Check sheet for the modelled part. Datum: model origin and axes. Units: mm. A direction names the side the tool comes from. Give positions to 0.01 mm unless a question says otherwise; leave off trailing zeros. Order: outer loops, then holes, each group sorted by start corner. A loop starts at its lowest first (then second) coordinate and runs counter-clockwise, first axis right, second up.
from build123d import *

# Parameters (mm, degrees)
SKETCH1_W           = 25
SKETCH1_H           = 25
SKETCH1_W_2         = 20
SKETCH1_H_2         = 20
BOSS_EXTRUDE1_DEPTH = 45
BOSS_EXTRUDE4_DEPTH = 45
FILLET2_R           = 2


with BuildPart() as part:
    # Sketch1 → Boss-Extrude1 (new body)
    with BuildSketch(Plane(origin=(0, 0, 0), x_dir=(1, 0, 0), z_dir=(0, 1, 0))):
        with Locations((12.5, 12.5)):
            Rectangle(SKETCH1_W, SKETCH1_H)
        with Locations((12.5, 12.5)):
            Rectangle(SKETCH1_W_2, SKETCH1_H_2, mode=Mode.SUBTRACT)
    extrude(amount=BOSS_EXTRUDE1_DEPTH)

    # Sketch3 → Boss-Extrude4 (add, through all)
    with BuildSketch(Plane.XZ):
        Polygon((22.5, -2.5), (12.5, -23.5), (2.5, -2.5), (4.404761905, -2.5), (12.5, -19.5), (20.595238095, -2.5), align=None)
    extrude(amount=-BOSS_EXTRUDE4_DEPTH)

    # Fillet2
    fillet2_edges = [part.edges().sort_by_distance(p)[0] for p in [
        (2.5, 22.5, -22.5),
        (22.5, 22.5, -22.5),
    ]]
    fillet(fillet2_edges, radius=FILLET2_R)


solid = part.part
1) Material ranges on L1, parallel to X at y = 28, z = -19.25; L2, parallel to Z at x = 15.75, y = 16.5 (3 decimals); L3, parallel to X at y = 5, z = -4, recorded low to high.
Recorded:
L1: x = 0 to 2.5, 10.48 to 12.38, 12.62 to 14.52, 22.5 to 25
L2: z = -25 to -22.5, -16.675 to -12.675, -2.5 to 0
L3: x = 0 to 2.5, 3.21 to 5.12, 19.88 to 21.79, 22.5 to 25
2) Set-up check for faces 5 (the face through (8.396, 22.185, -10.881)), 6 (the face through (10, 0, -15)): record each of +Z, -Z, +X, -X, +Y, -Y from which the full face is reachable in a straight line by a thin tool's end or side.
Recorded:
face 5: +Y, -Y
face 6: +Z, -Z, +X, -X, -Y
3) Section check A-A, the plane x = 19.5. Record the cut outline in (y, z).
Recorded:
outline: (0, -25) - (45, -25) - (45, -22.5) - (0, -22.5) - close; (0, -8.8) - (45, -8.8) - (45, -4.8) - (0, -4.8) - close; (0, -2.5) - (45, -2.5) - (45, 0) - (0, 0) - close
4) Section check C-C, the plane y = 4.5. Record the cut outline in (x, z), then the cut area to 3 significant figures.
Recorded:
outline: (0, -25) - (25, -25) - (25, 0) - (0, 0) - close; hole (2.5, -20.5) arc R2 ccw to (4.5, -22.5) - (12.02, -22.5) - (2.5, -2.5) - close; hole (4.4, -2.5) - (12.5, -19.5) - (20.6, -2.5) - close; hole (12.98, -22.5) - (20.5, -22.5) arc R2 ccw to (22.5, -20.5) - (22.5, -2.5) - close
area: 299 mm2
5) Draft check along Z on faces 1 (the face through (22.5, 22, -11)), 2 (the face through (12, 22, -2.5)), 3 (the face through (12, 22, -25)), 4 (the face through (25, 22, -12)). Enter one of: +Z half, -Z half, draft (parallel to the pull), parting line (faces both ways), or undercut.
Recorded:
face 1: undercut
face 2: undercut
face 3: -Z half
face 4: draft
6) Section check B-B, the plane z = -7.5. Record the cut outline in (x, y).
Recorded:
outline: (0, 0) - (2.5, 0) - (2.5, 45) - (0, 45) - close; (4.88, 0) - (6.79, 0) - (6.79, 45) - (4.88, 45) - close; (18.21, 0) - (20.12, 0) - (20.12, 45) - (18.21, 45) - close; (22.5, 0) - (25, 0) - (25, 45) - (22.5, 45) - close
